The model under review builds one solid part; all positions refer to its coordinate system, in mm. Round coordinates to 2 decimals unless told otherwise and drop trailing zeros. Write each loop counter-clockwise with the first axis right and the second up, starting at its lowest first coordinate (ties: lowest second). Pieces come first, ordered by that corner, then holes. Notation, with made-up numbers: (14.25, 62) - (71.25, 62) arc R22 ccw to (71.25, 88) - close; hole circle Ø7 at (7, 88). An arc over 180 degrees is marked (long way). One line per question, with ' | ' between items. Start each with the question number.
```python
from build123d import *

# Parameters (mm, degrees)
BOSS_EXTRUDE1_DEPTH      = 5
BOSS_EXTRUDE1_DEPTH_BACK = 5
SKETCH1_R                = 7.5


with BuildPart() as part:
    # Sketch1 → Boss-Extrude1 (new, two sides: drawn at the far end of the back side and taken through both)
    with BuildSketch(Plane.XY.offset(-BOSS_EXTRUDE1_DEPTH_BACK)):
        Polygon((-90, -50), (-48.817479436, -50), (90, 27.120821909), (90, 50), (-90, 50), align=None)
        with Locations((-70, 27.120821909)):
            Circle(SKETCH1_R, mode=Mode.SUBTRACT)
        with Locations((-70, -30)):
            Circle(SKETCH1_R, mode=Mode.SUBTRACT)
    extrude(amount=BOSS_EXTRUDE1_DEPTH + BOSS_EXTRUDE1_DEPTH_BACK)


solid = part.part
```
1. Clearance check with flat-ended pins moving along their axes: P1, Ø1, axis at y = -16.5, z = 0.5, coming from the +X side; P2, Ø19.5, axis at x = -70, y = 27.12, coming from the +Z side; P3, Ø6, axis at y = 14, z = 2, coming from the +X side. State where each tip first meets the part, or that it passes through.
2. Add section A-A, the plane x = -70. Write out the cut boundary in (y, z), then the cut area to 3 significant figures.
3. Wall thickness on line 1 along Y through (x, z) = (-70, -2.25); line 2 along X through (y, z) = (24, -3); line 3 along X through (y, z) = (-29.5, 1.5): over which ranges is each line inside the solid? List them lowest first. Write a range as [from, to].
4. Add section C-C, the plane y = -32. Write out the cut boundary in (x, z), then the cut area to 3 significant figures.
5. Add section D-D, the plane x = 36. Write out the cut boundary in (y, z).
6. Add section B-B, the plane z = 2.25. Write out the cut boundary in (x, y), then the cut area to 3 significant figures.
7. The part is to be moulded in two halves that separate along Y. For faces 1 (the face through (1, 50, 0)), 2 (the face through (19.62, -11.98, -0.07)), 3 (the face through (-77.493, 27.451, -0.07)), 4 (the face through (-90, 1, 0)), say which applies: pulls with the +Y half, pulls with the -Y half, needs draft (parallel to the pull), parting line crosses it, or undercut.
Geometry check:
1) P1: stops at x = 12.38 | P2: stops at z = 5 | P3: stops at x = 71.78
2) outline: (-50, -5) - (-37.5, -5) - (-37.5, 5) - (-50, 5) - close; (-22.5, -5) - (19.62, -5) - (19.62, 5) - (-22.5, 5) - close; (34.62, -5) - (50, -5) - (50, 5) - (34.62, 5) - close | area: 700 mm2
3) line 1: y = [-50, -37.5], [-22.5, 19.62], [34.62, 50] | line 2: x = [-90, -76.82], [-63.18, 84.38] | line 3: x = [-90, -77.48], [-62.52, -11.92]
4) outline: (-90, -5) - (-77.23, -5) - (-77.23, 5) - (-90, 5) - close; (-62.77, -5) - (-16.42, -5) - (-16.42, 5) - (-62.77, 5) - close | area: 591 mm2
5) outline: (-2.88, -5) - (50, -5) - (50, 5) - (-2.88, 5) - close
6) outline: (-90, -50) - (-48.82, -50) - (90, 27.12) - (90, 50) - (-90, 50) - close; hole circle Ø15 at (-70, -30); hole circle Ø15 at (-70, 27.12) | area: 12,300 mm2
7) face 1: pulls with the +Y half | face 2: pulls with the -Y half | face 3: undercut | face 4: needs draft
